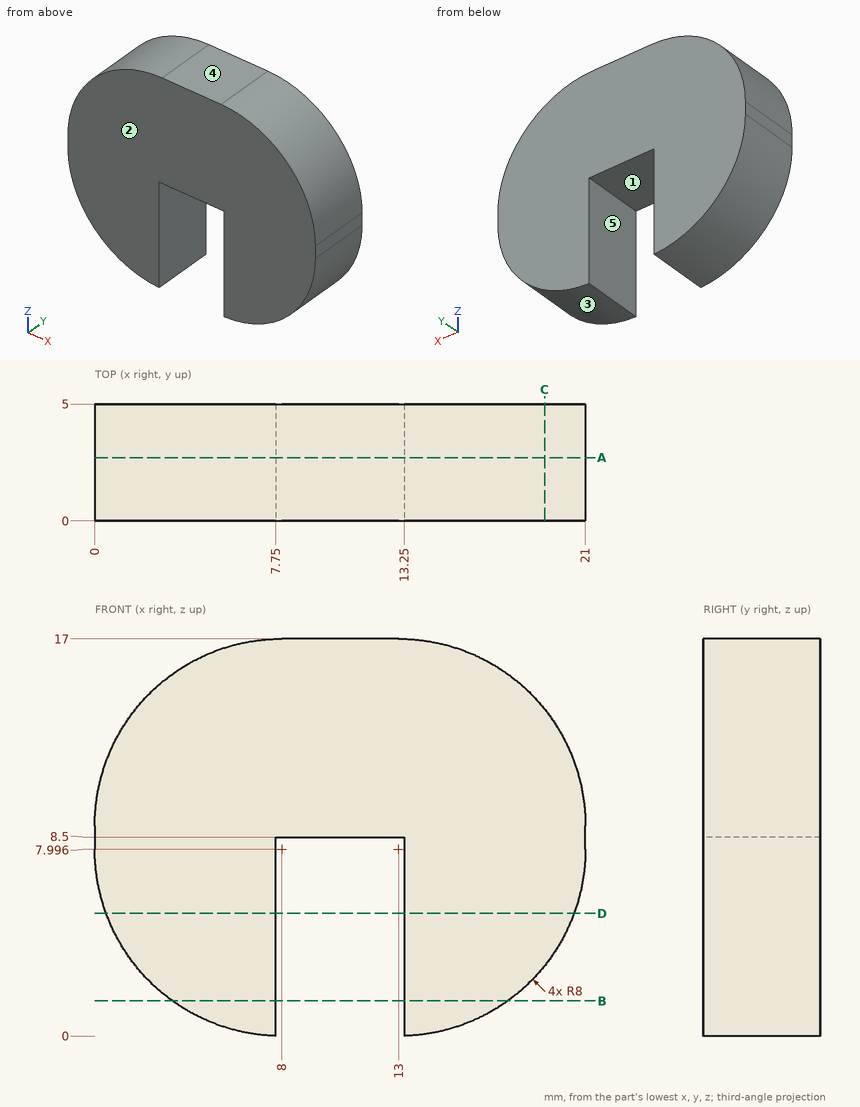
Geometry: see drawing. Coordinates: mm, zero at the bounding-box minimum. A direction names the side the tool comes from. Round coordinates to 2 decimals unless told otherwise and drop trailing zeros. Loops run counter-clockwise (first coordinate to the right, second up) from the corner with the lowest first, then second, coordinate; pieces in that order, holes last.
(1) Pull-direction query (X, two-part tool) for the marked faces 3, 4 and 5; classes: +X half, -X half, draft (parallel to the pull), parting line (faces both ways), or undercut.
From the geometry:
face 3: +X half
face 4: draft
face 5: undercut
(2) Section query D-D (z = 5.25). Output: boundary loops of the cut face in (x, y), and give its area (3 significant figures).
From the geometry:
outline: (0.49, 0) - (7.75, 0) - (7.75, 5) - (0.49, 5) - close; (13.25, 0) - (20.51, 0) - (20.51, 5) - (13.25, 5) - close
area: 72.6 mm2
(3) Section query B-B (z = 1.5). Output: boundary loops of the cut face in (x, y).
From the geometry:
outline: (3.33, 0) - (7.75, 0) - (7.75, 5) - (3.33, 5) - close; (13.25, 0) - (17.67, 0) - (17.67, 5) - (13.25, 5) - close
(4) Section query C-C (x = 19.25). Output: boundary loops of the cut face in (y, z).
From the geometry:
outline: (0, 3) - (5, 3) - (5, 13.99) - (0, 13.99) - close
(5) Contact query for flat-ended pins moving along their axis: pin 1 Ø3 at (y, z) = (0.5, 10.5) entering from -X; pin 2 Ø1.5 at (x, y) = (9.5, 2) entering from -Z; pin 3 Ø1 at (x, y) = (6, 1.5) entering from -Z. Output: stop coordinate, or through.
From the geometry:
pin 1: stops at x = 0
pin 2: stops at z = 8.5
pin 3: stops at z = 0.14
(6) Material intervals for probe 1 along X at (y, z) = (1.75, 8); probe 2 along Z at (x, y) = (8, 1.7); probe 3 along X at (y, z) = (3.65, 1), sorted ascending.
From the geometry:
probe 1: x = 0 to 7.75, 13.25 to 21
probe 2: z = 8.5 to 17
probe 3: x = 4.12 to 7.75, 13.25 to 16.88
(7) Section query A-A (y = 2.7). Output: boundary loops of the cut face in (x, z).
From the geometry:
outline: (0, 8) arc R8 ccw to (7.75, 0) - (7.75, 8.5) - (13.25, 8.5) - (13.25, 0) arc R8 ccw to (21, 8) - (21, 9) arc R8 ccw to (13, 17) - (8, 17) arc R8 ccw to (0, 9) - close
(8) Access query for the marked faces 1 and 2. Directions: +Z, -Z, +X, -X, +Y, -Y. A direction counts if a zero-diameter tool reaches every point of the face in a straight line with its end or side. Return the directions, or none.
From the geometry:
face 1: -Z, +Y, -Y
face 2: +Z, -Z, +X, -X, -Y
